Here's how the part is built. I have some questions about the finished solid (model axes, mm). A direction names the side the tool comes from. Round coordinates to 2 decimals unless told otherwise and drop trailing zeros. Loops run counter-clockwise (first coordinate to the right, second up) from the corner with the lowest first, then second, coordinate; pieces in that order, holes last. Notation, with made-up numbers: M 42,33 L 81,33 A22 ccw 81,48 Z; hole C 71,-38 d2. An arc over 180 degrees is marked long. Answer as CSV lines item,"result".
```python
from build123d import *

# Parameters (mm, degrees)
SKETCH1_W           = 8.5
SKETCH1_H           = 8.5
BOSS_EXTRUDE1_DEPTH = 300
SKETCH2_W           = 7
SKETCH2_H           = 7
CUT_EXTRUDE2_DEPTH  = 175
SKETCH4_R           = 2
CUT_EXTRUDE4_DEPTH  = 10
SKETCH6_W           = 7
SKETCH6_H           = 7
CUT_EXTRUDE5_DEPTH  = 26
SKETCH7_R           = 2
CUT_EXTRUDE6_DEPTH  = 26
SKETCH8_W           = 7
SKETCH8_H           = 7
CUT_EXTRUDE7_DEPTH  = 85
BOSS_EXTRUDE2_START = -7
SKETCH9_W           = 7
SKETCH9_H           = 7
SKETCH9_R           = 2
BOSS_EXTRUDE2_DEPTH = 7


with BuildPart() as part:
    # Sketch1 → Boss-Extrude1 (new body)
    with BuildSketch(Plane(origin=(0, 0, 0), x_dir=(1, 0, 0), z_dir=(0, 1, 0))):
        with Locations((4.25, 4.25)):
            Rectangle(SKETCH1_W, SKETCH1_H)
    extrude(amount=BOSS_EXTRUDE1_DEPTH)

    # Sketch2 → Cut-Extrude2 (cut)
    with BuildSketch(Plane(origin=(0, 33, 0), x_dir=(-1, 0, 0), z_dir=(0, -1, 0))):
        with Locations((-5, 3.5)):
            Rectangle(SKETCH2_W, SKETCH2_H)
    extrude(amount=-CUT_EXTRUDE2_DEPTH, mode=Mode.SUBTRACT)

    # Sketch4 → Cut-Extrude4 (cut)
    with BuildSketch(Plane.XZ.offset(-208)):
        with Locations(Location((5, -3.5, 0), (0, 0, 270))):
            Circle(SKETCH4_R)
    extrude(amount=-CUT_EXTRUDE4_DEPTH, mode=Mode.SUBTRACT)

    # Sketch6 → Cut-Extrude5 (cut)
    with BuildSketch(Plane.XZ):
        with Locations((5, -3.5)):
            Rectangle(SKETCH6_W, SKETCH6_H)
    extrude(amount=-CUT_EXTRUDE5_DEPTH, mode=Mode.SUBTRACT)

    # Sketch7 → Cut-Extrude6 (cut)
    with BuildSketch(Plane.XZ.offset(-26)):
        with Locations(Location((5, -3.5, 0), (0, 0, 270))):
            Circle(SKETCH7_R)
    extrude(amount=-CUT_EXTRUDE6_DEPTH, mode=Mode.SUBTRACT)

    # Sketch8 → Cut-Extrude7 (cut)
    with BuildSketch(Plane(origin=(0, 300, 0), x_dir=(1, 0, 0), z_dir=(0, 1, 0))):
        with Locations((5, 3.5)):
            Rectangle(SKETCH8_W, SKETCH8_H)
    extrude(amount=-CUT_EXTRUDE7_DEPTH, mode=Mode.SUBTRACT)

    # Sketch9 → Boss-Extrude2 (add)
    with BuildSketch(Plane(origin=(0, 300, 0), x_dir=(1, 0, 0), z_dir=(0, 1, 0)).offset(BOSS_EXTRUDE2_START)):
        with Locations((5, 3.5)):
            Rectangle(SKETCH9_W, SKETCH9_H)
        with Locations(Location((5, 3.5, 0), (0, 0, 90))):
            Circle(SKETCH9_R, mode=Mode.SUBTRACT)
    extrude(amount=BOSS_EXTRUDE2_DEPTH)


solid = part.part
```
1. If I drill on line 1 (Y direction, x = 2.5, z = -4); line 2 (X direction, y = 29.5, z = -3.5); line 3 (Z direction, x = 5, y = 295.25), over which ranges is the centre line in solid material (lowest first)? Write a range as [from, to].
Evaluation:
line 1,"y = [26, 33], [208, 215], [293, 300]"
line 2,"x = [0, 3], [7, 8.5]"
line 3,"z = [-8.5, -5.5], [-1.5, 0]"
2. I want a section at C-C, the plane y = 169.5. Please give me the cut outline in (x, z).
Evaluation:
outline,"M 0,-8.5 L 8.5,-8.5 L 8.5,-7 L 1.5,-7 L 1.5,0 L 0,0 Z"
3. We'd pull the mould along Y, two halves only. Please class faces 1 (the flat face through (1, 0, -6)), 2 (the flat face through (1.5, 13, -4)), 3 (the flat face through (3, 215, -2)), 4 (the flat face through (3, 300, -5)): pulls with the +Y half, pulls with the -Y half, needs draft (parallel to the pull), parting line crosses it, or undercut.
Evaluation:
face 1,"pulls with the -Y half"
face 2,"needs draft"
face 3,"undercut"
face 4,"pulls with the +Y half"
4. I want a section at B-B, the plane x = 5. Please give me the cut outline in (y, z).
Evaluation:
outline,"M 0,-8.5 L 300,-8.5 L 300,-5.5 L 293,-5.5 L 293,-7 L 215,-7 L 215,-5.5 L 208,-5.5 L 208,-7 L 33,-7 L 33,-5.5 L 26,-5.5 L 26,-7 L 0,-7 Z; M 26,-1.5 L 33,-1.5 L 33,0 L 26,0 Z; M 208,-1.5 L 215,-1.5 L 215,0 L 208,0 Z; M 293,-1.5 L 300,-1.5 L 300,0 L 293,0 Z"
5. For P1, Ø2, axis at y = 151.5, z = -2, coming from the +X side; P2, Ø3.5, axis at x = 3.5, z = -2.5, coming from the -Y side; P3, Ø3.5, axis at x = 5, z = -3.5, coming from the -Y side; P4, Ø2, axis at x = 6.5, y = 255.5, coming from the +Z side, each with a flat end and sliding along its axis, tell me the tip position at first contact or that it passes through.
Evaluation:
P1,"stops at x = 1.5"
P2,"stops at y = 26"
P3,"passes through"
P4,"stops at z = -7"
6. I want a section at A-A, the plane z = -3.5. Please give me the cut outline in (x, y), and give its area (3 significant figures).
Evaluation:
outline,"M 0,0 L 1.5,0 L 1.5,26 L 3,26 L 3,33 L 1.5,33 L 1.5,208 L 3,208 L 3,215 L 1.5,215 L 1.5,293 L 3,293 L 3,300 L 0,300 Z; M 7,26 L 8.5,26 L 8.5,33 L 7,33 Z; M 7,208 L 8.5,208 L 8.5,215 L 7,215 Z; M 7,293 L 8.5,293 L 8.5,300 L 7,300 Z"
area,"513 mm²"
7. Which directions (+Z, -Z, +X, -X, +Y, -Y) give clear straight access to the entire face, cutting with the end or side of a thin tool? Please do faces 5 (the flat face through (3, 26, -5)), 6 (the flat face through (1, 116, 0)), 7 (the flat face through (5, 255, -7)).
Evaluation:
face 5,"+Z, +X, -Y"
face 6,"+Z, +X, -X, +Y, -Y"
face 7,"+Z, +X"
